Autodesk Inventor part; units mm, degrees
ref_plane "YZ Plane" through (0, 0, 0) normal (1, 0, 0) x (0, 1, 0)
ref_plane "XZ Plane" through (0, 0, 0) normal (0, 1, 0) x (-1, 0, 0)
ref_plane "XY Plane" through (0, 0, 0) normal (0, 0, 1) x (1, 0, 0)
sketch "Szkic1" plane through (0, 0, 0) normal (0, 0, 1) x (1, 0, 0)
  line L0 (0, 0) -> (40, 0)
  line L1 (40, 0) -> (40, 110)
  line L2 (40, 110) -> (0, 110)
  line L3 (0, 110) -> (0, 0)
  circle A0 centre (20, 110) radius 11.5
  circle A1 centre (20, 110) radius 20
  dimension "d0" = 40
  dimension "d1" = 110
  dimension "d2" = 23
extrude "Wyciągnięcie proste1" add sketch "Szkic1" along normal blind 25 contours L3 A1 L1 L0 | A1 L2 A0 | L2 A0 A1
sketch "Szkic2" plane through (0, 0, 25) normal (0, 0, 1) x (1, 0, 0)
  line L0 (0, 110) -> (0, 0)
  line L1 (0, 0) -> (0, 23)
  line L2 (0, 23) -> (40, 23)
  line L3 (40, 0) -> (40, 110)
  line L4 (40, 23) -> (40, 0)
  line L5 (40, 0) -> (0, 0)
  dimension "d5" = 23
  dimension "d6" = 40
extrude "Wyciągnięcie proste2" add sketch "Szkic2" along normal blind 32
properties part number "Podstawa"
Build history of the part. All positions in model axes, mm. A direction names the side the tool comes from. Give positions to 0.01 mm unless a question says otherwise; leave off trailing zeros. Loops run counter-clockwise (first coordinate to the right, second up) from the corner with the lowest first, then second, coordinate; pieces in that order, holes last. Notation, with made-up numbers: (-27, 73) -> (30, 73) arc R23 cw to (30, 96) -> close; hole circle Ø9 at (-8.75, 18). An arc over 180 degrees is marked (long way). One line per question, with ' | ' between items. Start each with the question number.
1) Cut at D-D (x = 28). Give the cut face in (y, z).
2) Cut at C-C (z = 4.5). Give the cut face in (x, y).
3) Cut at B-B (y = 112.5). Give the cut face in (x, z).
4) Probe L1, parallel to X at y = 110, z = 11.75; L2, parallel to Y at x = 20, z = 17; L3, parallel to Z at x = 13, y = 75. List the from-to ranges inside material, lowest first.
5) Pin check, flat tips, straight feed: pin 1 (6 mm diameter, centred on x = 35.5, y = 63.5, fed in from +Z); pin 2 (5 mm diameter, centred on x = 35, z = 27.5, fed in from -Y). Stop position of each tip, or through.
6) Cut at A-A (x = 20). Give the cut face in (y, z).
7) Two-plate mould, pull along X, no slides. Class faces 3 (the flat face through (20, 77, 25)), 4 (the flat face through (40, 42, 15)), 5 (the cylindrical face through (30.97, 106.55, 12.32)): released by +X, released by -X, zero draft, split by the parting line, or undercut.
8) 3-axis set-ups, long thin cutter, end or side, ignore diameter. For faces 1 (the flat face through (20, 23, 41)), 2 (the cylindrical face through (20, 130, 12)): which of +Z, -Z, +X, -X, +Y, -Y reach the whole face in a straight line?
Return value:
1) outline: (0, 0) -> (101.74, 0) -> (101.74, 25) -> (23, 25) -> (23, 57) -> (0, 57) -> close; (118.26, 0) -> (128.33, 0) -> (128.33, 25) -> (118.26, 25) -> close
2) outline: (0, 0) -> (40, 0) -> (40, 110) arc R20 ccw to (0, 110) -> close; hole circle Ø23 at (20, 110)
3) outline: (0.16, 0) -> (8.78, 0) -> (8.78, 25) -> (0.16, 25) -> close; (31.22, 0) -> (39.84, 0) -> (39.84, 25) -> (31.22, 25) -> close
4) L1: 0 to 8.5, 31.5 to 40 | L2: 0 to 98.5, 121.5 to 130 | L3: 0 to 25
5) pin 1: z = 25 | pin 2: y = 0
6) outline: (0, 0) -> (98.5, 0) -> (98.5, 25) -> (23, 25) -> (23, 57) -> (0, 57) -> close; (121.5, 0) -> (130, 0) -> (130, 25) -> (121.5, 25) -> close
7) face 3: zero draft | face 4: released by +X | face 5: undercut
8) face 1: +Z, +X, -X, +Y | face 2: +Z, -Z, +Y
